Verification items for this drawing (mm, ordinates from the low corner). A direction names the side the tool comes from. Coordinates: 2 decimals unless noted, no trailing zeros. Write each loop counter-clockwise with the first axis right and the second up, starting at its lowest first coordinate (ties: lowest second). Pieces come first, ordered by that corner, then holes.
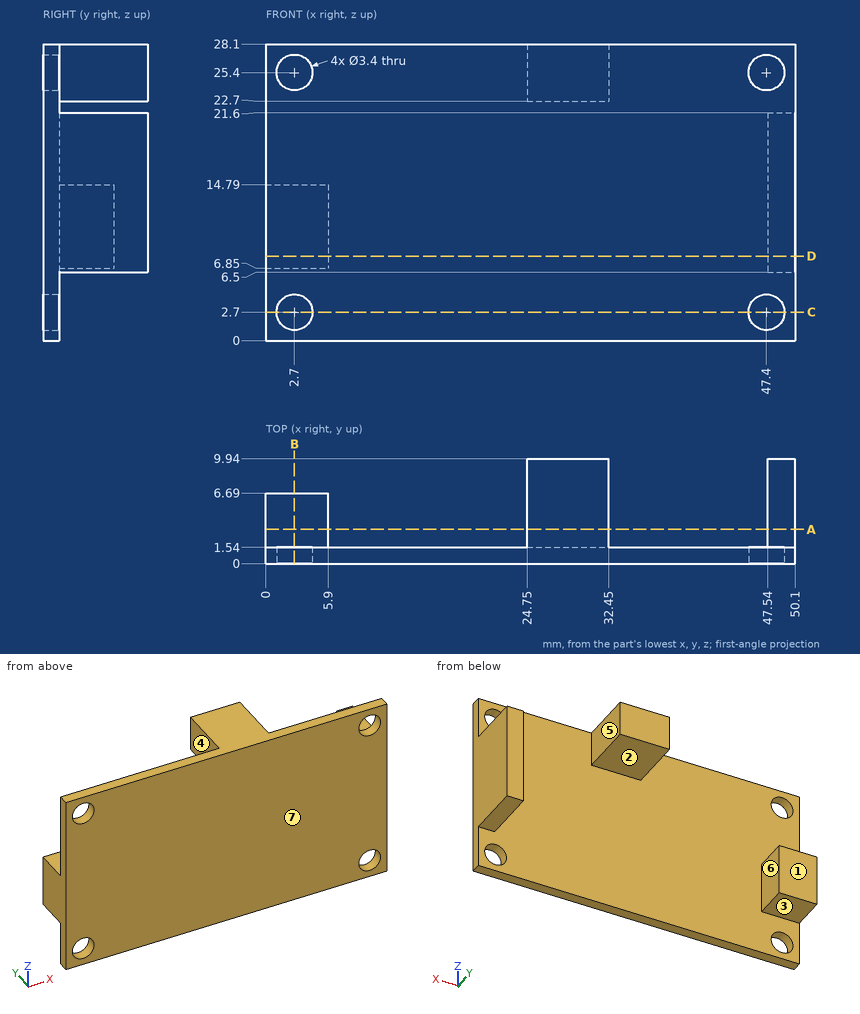
1. Sectioned sample at C-C, the plane z = 2.7. Record the boundary of the cut face in (x, y).
Computed values:
outline: (0, 0) - (1, 0) - (1, 1.54) - (0, 1.54) - close; (4.4, 0) - (45.7, 0) - (45.7, 1.54) - (4.4, 1.54) - close; (49.1, 0) - (50.1, 0) - (50.1, 1.54) - (49.1, 1.54) - close
2. Sectioned sample at B-B, the plane x = 2.7. Record the boundary of the cut face in (y, z).
Computed values:
outline: (0, 0) - (1.54, 0) - (1.54, 1) - (0, 1) - close; (0, 4.4) - (1.54, 4.4) - (1.54, 6.85) - (6.69, 6.85) - (6.69, 14.79) - (1.54, 14.79) - (1.54, 23.7) - (0, 23.7) - close; (0, 27.1) - (1.54, 27.1) - (1.54, 28.1) - (0, 28.1) - close
3. Sectioned sample at D-D, the plane z = 8. Record the boundary of the cut face in (x, y).
Computed values:
outline: (0, 0) - (50.1, 0) - (50.1, 9.94) - (47.54, 9.94) - (47.54, 1.54) - (5.9, 1.54) - (5.9, 6.69) - (0, 6.69) - close
4. Access from +Z, -Z, +X, -X, +Y, -Y to the whole of each face (thin tool, end or side, straight path). Record for the marked faces 1, 2 and 3.
Computed values:
face 1: +Z, -Z, -X, +Y
face 2: -Z, +X, -X, +Y
face 3: -Z, -X, +Y
5. Thickness scan on line 1 along X through (y, z) = (0.3, 25.4); line 2 along X through (y, z) = (1.5, 4); line 3 along X through (y, z) = (5.5, 12.25). Record the ranges inside material, lowest first.
Computed values:
line 1: x = 0 to 1, 4.4 to 45.7, 49.1 to 50.1
line 2: x = 0 to 1.6, 3.8 to 46.3, 48.5 to 50.1
line 3: x = 0 to 5.9, 47.54 to 50.1
6. Gauge pin test, flat ends, axial feed: pin 1 Ø2.5 at (y, z) = (6.5, 25.5) entering from -X; pin 2 Ø2 at (x, z) = (47.4, 25.4) entering from -Y; pin 3 Ø8 at (x, z) = (37.5, 15) entering from -Y; pin 4 Ø1.3 at (x, y) = (49.5, 8) entering from +Z. Record the tip position at first contact, or that the pin passes through.
Computed values:
pin 1: stops at x = 24.75
pin 2: passes through
pin 3: stops at y = 0
pin 4: stops at z = 21.6
7. Draft check along X on the marked faces 4, 5, 6 and 7. Enter one of: released by +X, released by -X, zero draft, split by the parting line, or undercut.
Computed values:
face 4: released by -X
face 5: released by +X
face 6: undercut
face 7: zero draft
8. Sectioned sample at A-A, the plane y = 3.25. Record the boundary of the cut face in (x, z).
Computed values:
outline: (0, 6.85) - (5.9, 6.85) - (5.9, 14.79) - (0, 14.79) - close; (24.75, 22.7) - (32.45, 22.7) - (32.45, 28.1) - (24.75, 28.1) - close; (47.54, 6.5) - (50.1, 6.5) - (50.1, 21.6) - (47.54, 21.6) - close
